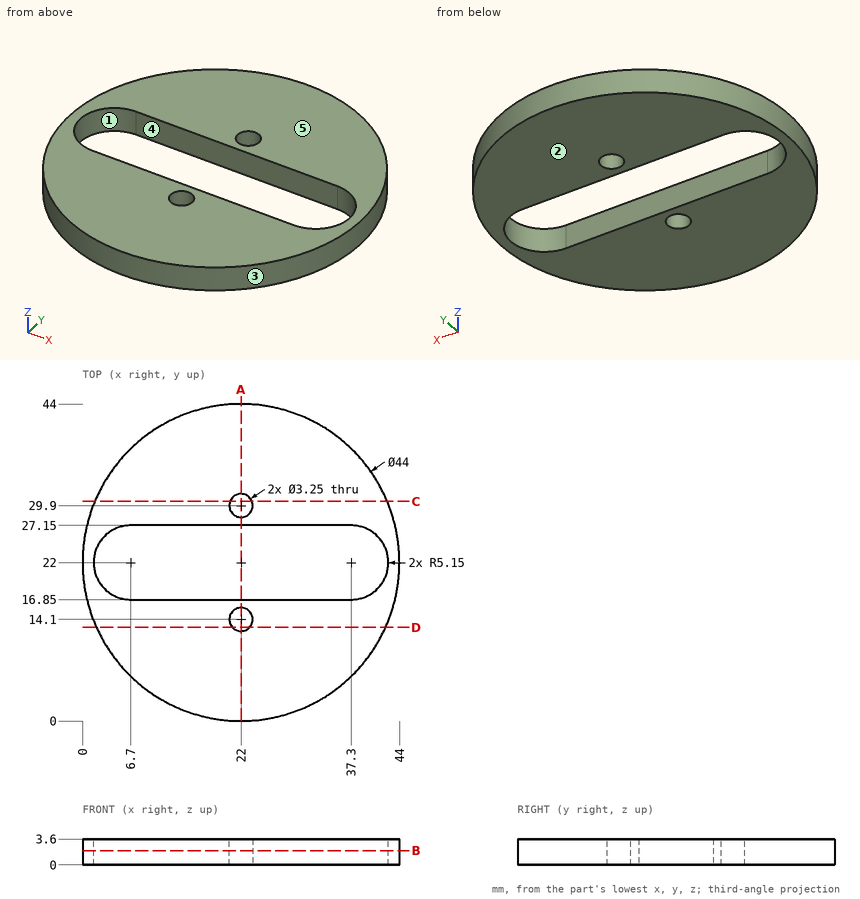
Part print with two shaded views. Sizes in mm from the minimum x, y, z corner. A direction names the side the tool comes from. Give positions to 0.01 mm unless a question says otherwise; leave off trailing zeros. Loops run counter-clockwise (first coordinate to the right, second up) from the corner with the lowest first, then second, coordinate; pieces in that order, holes last. Notation, with made-up numbers: (47, 17.25) -> (89, 17.25) arc R8 ccw to (89, 23.25) -> close; hole circle Ø8 at (11, 85.25). An arc over 180 degrees is marked (long way). One line per question, with ' | ' between items.
Q1. Pull direction Y, two halves, no side cores. Call the marked faces 1, 2 and 3: pulls with the +Y half, pulls with the -Y half, needs draft (parallel to the pull), parting line crosses it, or undercut.
Filled sheet:
face 1: undercut | face 2: needs draft | face 3: parting line crosses it
Q2. Cut at A-A, the plane x = 22. Write the cut outline in (y, z) (3 decimals), plus the area to 3 significant figures.
Filled sheet:
outline: (0, 0) -> (12.475, 0) -> (12.475, 3.6) -> (0, 3.6) -> close; (15.725, 0) -> (16.85, 0) -> (16.85, 3.6) -> (15.725, 3.6) -> close; (27.15, 0) -> (28.275, 0) -> (28.275, 3.6) -> (27.15, 3.6) -> close; (31.525, 0) -> (44, 0) -> (44, 3.6) -> (31.525, 3.6) -> close | area: 97.9 mm²
Q3. Tool access for the marked faces 4 and 5: list every direction of +Z, -Z, +X, -X, +Y, -Y with a clear straight run to the whole face (end or side of a thin tool).
Filled sheet:
face 4: +Z, -Z | face 5: +Z, +X, -X, +Y, -Y
Q4. Cut at D-D, the plane y = 13. Write the cut outline in (x, z), plus the area to 3 significant figures.
Filled sheet:
outline: (1.93, 0) -> (20.8, 0) -> (20.8, 3.6) -> (1.93, 3.6) -> close; (23.2, 0) -> (42.07, 0) -> (42.07, 3.6) -> (23.2, 3.6) -> close | area: 136 mm²
Q5. Cut at C-C, the plane y = 30.5. Write the cut outline in (x, z).
Filled sheet:
outline: (1.71, 0) -> (20.49, 0) -> (20.49, 3.6) -> (1.71, 3.6) -> close; (23.51, 0) -> (42.29, 0) -> (42.29, 3.6) -> (23.51, 3.6) -> close
Q6. Drop flat-ended pins along their axis: pin 1 (2 mm diameter, centred on x = 38.5, y = 5, fed in from +Z); pin 2 (1.8 mm diameter, centred on x = 25, z = 1, fed in from -Y). Give the stop position or say it passes through.
Filled sheet:
pin 1: passes through | pin 2: stops at y = 0.1
Q7. Cut at B-B, the plane z = 2. Write the cut outline in (x, y) (3 decimals).
Filled sheet:
outline: circle Ø44 at (22, 22); hole (6.7, 16.85) -> (37.3, 16.85) arc R5.15 ccw to (37.3, 27.15) -> (6.7, 27.15) arc R5.15 ccw to start; hole circle Ø3.25 at (22, 14.1); hole circle Ø3.25 at (22, 29.9)
Q8. Drill centre lines: line 1 along Y through (x, z) = (22, 2.4) (3 decimals); line 2 along Y through (x, z) = (20, 1.6); line 3 along X through (y, z) = (30.5, 2.8). Where is each one in solid material? Low to high. Write a range as [from, to].
Filled sheet:
line 1: y = [0, 12.475], [15.725, 16.85], [27.15, 28.275], [31.525, 44] | line 2: y = [0.09, 16.85], [27.15, 43.91] | line 3: x = [1.71, 20.49], [23.51, 42.29]
